```python
from build123d import *

# Parameters (mm, degrees)
SKETCH001_R        = 4.7
PAD_DEPTH          = 4
SKETCH003_R        = 2.55
POCKET_DEPTH       = 5
POLARPATTERN_COUNT = 6
SKETCH002_R        = 4.7
PAD001_DEPTH       = 48


with BuildPart() as part:
    # Sketch → Revolution (revolve)
    with BuildSketch(Plane.XZ):
        with BuildLine():
            Line((9.49, 51.71), (9.49, 103))
            Line((9.49, 103), (4.7, 103))
            Line((4.7, 103), (4.7, 0))
            Line((4.7, 0), (70, 0))
            Line((70, 0), (70, 0.2))
            Line((70, 0.2), (61, 0.2))
            ThreePointArc((9.49, 51.71), (24.57693, 15.28693), (61, 0.2))
        make_face()
    revolve(axis=Axis((0, 0, 0), (0, 0, 1)))

    # Sketch001 (on Face4 of Revolution) → Pad (new body)
    with BuildSketch(Plane(origin=(0, 0, 0), x_dir=(1, 0, 0), z_dir=(0, 0, -1))):
        Polygon((0, 100), (-86.60254, 50), (-86.60254, -50), (0, -100), (86.60254, -50), (86.60254, 50), align=None)
        Circle(SKETCH001_R, mode=Mode.SUBTRACT)
    extrude(amount=PAD_DEPTH)

    # Sketch003 → Pocket (cut)
    with BuildSketch(Plane(origin=(0, 0, -4), x_dir=(1, 0, 0), z_dir=(0, 0, -1))):
        with Locations((-57.807196, 60.125)):
            Circle(SKETCH003_R)
        with Locations((-40.486688, 70.125)):
            Circle(SKETCH003_R)
        with Locations((-23.16618, 80.125)):
            Circle(SKETCH003_R)
    pocket = extrude(amount=-POCKET_DEPTH, mode=Mode.SUBTRACT)

    # PolarPattern: Pocket ×6 about axis
    polarpattern_axis = Axis((0, 0, -4), (0, 0, -1))
    for i in range(1, POLARPATTERN_COUNT):
        add(pocket.rotate(polarpattern_axis, i * 360 / POLARPATTERN_COUNT), mode=Mode.SUBTRACT)

    # Sketch002 (on Face3 of Pad) → Pad001 (join)
    with BuildSketch(Plane(origin=(0, 0, 103), x_dir=(-1, 0, 0), z_dir=(0, 0, 1))):
        Polygon((0, 9.49), (-8.218581, 4.745), (-8.218581, -4.745), (0, -9.49), (8.218581, -4.745), (8.218581, 4.745), align=None)
        Circle(SKETCH002_R, mode=Mode.SUBTRACT)
    extrude(amount=PAD001_DEPTH)


solid = part.part
```
Source: CAD feature listing. Evaluate the final solid. Frame: model axes, mm. A direction names the side the tool comes from. Give positions to 0.01 mm unless a question says otherwise; leave off trailing zeros. Loops run counter-clockwise (first coordinate to the right, second up) from the corner with the lowest first, then second, coordinate; pieces in that order, holes last. Notation, with made-up numbers: (-40, 82) -> (-6, 82) arc R13 ccw to (-6, 105) -> close; hole circle Ø3 at (-13.75, 74.25). An arc over 180 degrees is marked (long way). Put each result on its own line as item: value. Start each with the question number.
1) Reachability of faces 4 (the face through (43.91, -74.65, -1.97)), 5 (the face through (-8.219, 0, 127)), 6 (the face through (4.4, -7.5, 103)), 7 (the face through (-4.167, -7.084, 126.664)), 8 (the face through (-58.139, 57.597, -2.028)) from +Z, -Z, +X, -X, +Y, -Y: full face, straight path, thin tool, end or side. Return the list, or none.
2) Draft query along Y for faces 1 (the face through (-2.057, -9.264, 77.714)), 2 (the face through (-1, 21, -4)), 3 (the face through (20.734, 80.891, -2.028)). Return one class per face: released by +Y, released by -Y, zero draft, split by the parting line, or undercut.
3) Contact query for flat-ended pins moving along their axis: P1, Ø10.5, axis at y = 0.5, z = 129, coming from the -X side; P2, Ø10, axis at x = -21.5, y = 14.5, coming from the +Z side; P3, Ø6.5, axis at x = -40.49, y = 70.13, coming from the +Z side; P4, Ø4, axis at x = 40.49, y = -70.13, coming from the +Z side. Output: stop coordinate, or through.
4) Material intervals for probe 1 along Y at (x, z) = (0, 124); probe 2 along Z at (x, y) = (66.5, 39.5); probe 3 along Z at (x, y) = (-20, -59), sorted ascending.
5) Cut plane B-B (z = 100.5). Return loops of the section in (x, y), then the cut area to 3 significant figures.
6) Cut plane A-A (z = 122.5). Return loops of the section in (x, y) (3 decimals), then the cut area to 3 significant figures.
7) Cut plane C-C (z = 45.5). Return loops of the section in (x, y), then the cut area to 3 significant figures.
Results are:
1. face 4: +Z, -Z, +X, -Y
1. face 5: +Z, -X, +Y, -Y
1. face 6: +Z, +X, -Y
1. face 7: +Z, -X, -Y
1. face 8: +Z, -Z
2. face 1: split by the parting line
2. face 2: zero draft
2. face 3: undercut
3. P1: stops at x = -8.22
3. P2: stops at z = 19.34
3. P3: stops at z = 0
3. P4: passes through
4. probe 1: y = -9.49 to -4.7, 4.7 to 9.49
4. probe 2: z = -4 to 0
4. probe 3: z = -4 to 0.2
5. outline: circle Ø18.98 at (0, 0); hole circle Ø9.4 at (0, 0)
5. area: 214 mm2
6. outline: (-8.219, -4.745) -> (0, -9.49) -> (8.219, -4.745) -> (8.219, 4.745) -> (0, 9.49) -> (-8.219, 4.745) -> close; hole circle Ø9.4 at (0, 0)
6. area: 165 mm2
7. outline: circle Ø19.73 at (0, 0); hole circle Ø9.4 at (0, 0)
7. area: 236 mm2
